Verification items for the finished model (mm, model axes). Face numbers are marked on the shaded views. Round coordinates to 2 decimals unless told otherwise and drop trailing zeros. Write each loop counter-clockwise with the first axis right and the second up, starting at its lowest first coordinate (ties: lowest second). Pieces come first, ordered by that corner, then holes. Notation, with made-up numbers: M 35,18 L 93,18 A21 cw 93,25 Z; hole C 18,-23.5 d5. An arc over 180 degrees is marked long. One line per question, with ' | ' between items.
from build123d import *

# Parameters (mm, degrees)
BOSS_EXTRUDE1_DEPTH = 6
BOSS_EXTRUDE2_DEPTH = 8
FILLET1_R           = 1


with BuildPart() as part:
    # Sketch1 → Boss-Extrude1 (new body)
    with BuildSketch(Plane.XY):
        with BuildLine():
            Line((-1.6, 0), (-2.1, 0))
            Line((-2.1, 0), (-3.835581375, -5.864960127))
            ThreePointArc((-3.835581375, -5.864960127), (0, -11), (3.835581375, -5.864960127))
            Line((3.835581375, -5.864960127), (2.1, 0))
            Line((2.1, 0), (1.6, 0))
            Line((1.6, 0), (1.6, -8))
            Line((1.6, -8), (0, -8))
            Line((0, -8), (-1.6, -8))
            Line((-1.6, -8), (-1.6, 0))
        make_face()
    extrude(amount=BOSS_EXTRUDE1_DEPTH)

    # Sketch2 → Boss-Extrude2 (add)
    with BuildSketch(Plane(origin=(0, -8, 0), x_dir=(1, 0, 0), z_dir=(0, 1, 0))):
        with BuildLine():
            Line((1.6, -6), (1.6, -3))
            ThreePointArc((1.6, -3), (0, -4.6), (-1.6, -3))
            Line((-1.6, -3), (-1.6, -6))
            Line((-1.6, -6), (1.6, -6))
        make_face()
        with BuildLine():
            Line((1.6, -3), (1.6, 0))
            Line((1.6, 0), (-1.6, 0))
            Line((-1.6, 0), (-1.6, -3))
            ThreePointArc((-1.6, -3), (0, -1.4), (1.6, -3))
        make_face()
    extrude(amount=BOSS_EXTRUDE2_DEPTH)

    # Fillet1
    # the kernel refuses this fillet: 1 mm, written as the material it takes off along each edge
    with BuildSketch(Plane(origin=(-4.6, 0, 0), x_dir=(0, 0, 1), z_dir=(1, 0, 0))) as fillet1_piece_1:
        with BuildLine():
            CenterArc((FILLET1_R, FILLET1_R), FILLET1_R, 180, 90)
            Line((0, FILLET1_R), (0, 0))
            Line((0, 0), (FILLET1_R, 0))
        make_face()
    extrude(amount=9.2, mode=Mode.SUBTRACT)
    with BuildSketch(Plane(origin=(2.1, 0, -1.867357153), x_dir=(-1, 0, 0), z_dir=(0, 0, 1))) as fillet1_piece_2:
        with BuildLine():
            CenterArc((FILLET1_R * 0.746942861214, FILLET1_R), FILLET1_R, 196.484740183, 73.515259817)
            Line((-FILLET1_R * 0.211952482607, FILLET1_R * 0.716240031718), (0, 0))
            Line((0, 0), (FILLET1_R * 0.746942861214, 0))
        make_face()
    extrude(amount=9.734714306, mode=Mode.SUBTRACT)
    with BuildSketch(Plane(origin=(-2.1, 0, -1.867357153), x_dir=(1, 0, 0), z_dir=(0, 0, 1))) as fillet1_piece_3:
        with BuildLine():
            CenterArc((FILLET1_R * 0.746942861214, -FILLET1_R), FILLET1_R, 90, 73.515259817)
            Line((-FILLET1_R * 0.211952482607, -FILLET1_R * 0.716240031718), (0, 0))
            Line((0, 0), (FILLET1_R * 0.746942861214, 0))
        make_face()
    extrude(amount=9.734714306, mode=Mode.SUBTRACT)
    with BuildSketch(Plane(origin=(4.6, 0, 6), x_dir=(0, -1, 0), z_dir=(-1, 0, 0))) as fillet1_piece_4:
        with BuildLine():
            CenterArc((FILLET1_R, -FILLET1_R), FILLET1_R, 90, 90)
            Line((0, -FILLET1_R), (0, 0))
            Line((0, 0), (FILLET1_R, 0))
        make_face()
    extrude(amount=9.2, mode=Mode.SUBTRACT)


solid = part.part
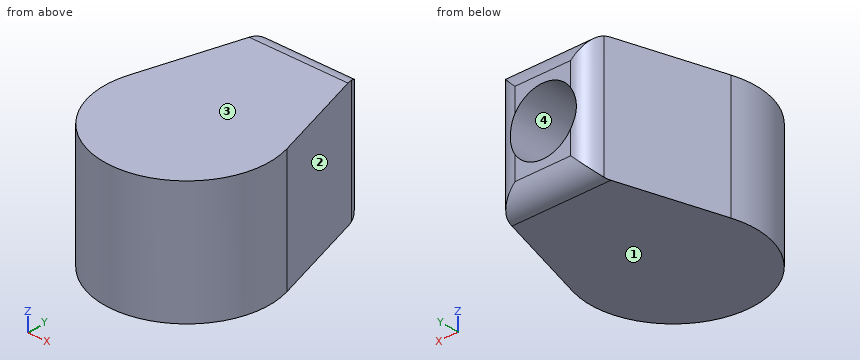
1. Section check B-B, the plane y = -7. Record the cut outline in (x, z).
Results:
outline: M -4,0 L 4,0 L 4,6 L -4,6 Z; hole C 0,3 d3.2
2. Thickness scan on line 1 (Z direction, x = 0, y = -2); line 2 (X direction, y = -6.75, z = 4.1); line 3 (X direction, y = -3.75, z = 4.2). Record the ranges inside material, lowest first.
Results:
line 1: z = 0 to 1.4, 4.6 to 6 | line 2: x = -3.99 to -1.16, 1.16 to 3.99 | line 3: x = -3.21 to -1.06, 1.06 to 3.21
3. Mould release check, pull along Z, two halves, no side actions. Record for the marked faces 1, 2, 3 and 4: pulls with the +Z half, pulls with the -Z half, needs draft (parallel to the pull), parting line crosses it, or undercut.
Results:
face 1: pulls with the -Z half | face 2: needs draft | face 3: pulls with the +Z half | face 4: undercut
4. Section check C-C, the plane z = 1.8. Record the cut outline in (x, y), then the cut area to 3 significant figures.
Results:
outline: M -3.84,-5.86 A4 ccw long 3.84,-5.86 L 2.31,-0.72 A1 ccw 1.35,0 L 1.06,0 L 1.06,-8 L -1.06,-8 L -1.06,0 L -1.35,0 A1 ccw -2.31,-0.72 Z | area: 51.8 mm2
5. Section check D-D, the plane z = 3. Record the cut outline in (x, y), then the cut area to 3 significant figures.
Results:
outline: M -3.84,-5.86 A4 ccw long 3.84,-5.86 L 2.31,-0.72 A1 ccw 1.6,-0.03 L 1.6,-8 L -1.6,-8 L -1.6,-0.03 A1 ccw -2.31,-0.72 Z | area: 43.1 mm2
6. Section check A-A, the plane x = 0. Record the cut outline in (y, z).
Results:
outline: M -11,0 L -1,0 A1 ccw 0,1 L 0,1.4 L -8,1.4 L -8,4.6 L 0,4.6 L 0,5 A1 ccw -1,6 L -11,6 Z
7. Go/stop test with flat-tipped pins: P1, Ø3, axis at y = -5, z = 1.5, coming from the +X side; P2, Ø1, axis at x = 0.5, z = 2.5, coming from the +Y side; P3, Ø2, axis at y = -3.5, z = 2, coming from the +X side. Record where each tip stops, or that it passes through.
Results:
P1: stops at x = 3.97 | P2: stops at y = -8 | P3: stops at x = 3.43
